Part model, mm, in its own coordinate system. A direction names the side the tool comes from. Round coordinates to 2 decimals unless told otherwise and drop trailing zeros. Write each loop counter-clockwise with the first axis right and the second up, starting at its lowest first coordinate (ties: lowest second). Pieces come first, ordered by that corner, then holes. Notation, with made-up numbers: M 83.25,48.5 L 108.25,48.5 A25 ccw 108.25,73.5 Z; hole C -26.5,0 d4. An arc over 180 degrees is marked long. Use one line per item in the form item = value. Start each with the question number.
Item 1: Cut at D-D, the plane z = 0. Give the cut face in (x, y).
Item 2: Cut at B-B, the plane z = -20.4. Give the cut face in (x, y).
Item 3: Which spindle directions (+Z, -Z, +X, -X, +Y, -Y) get a long thin tool onto all of the face, cutting with end or side? Do faces 1 (the face through (7.5, -17, -44)), 2 (the face through (-40, 0, 0)), 3 (the face through (40, 0, 0)), 4 (the face through (-43.7, 0.6, -20.9)), 5 (the face through (0, 0, 29)). Say none if no direction does.
Item 4: Mould opens along X. For faces 6 (the face through (38.9, 0.6, 19.6)), 7 (the face through (-1.352, 21.906, -4.292)), 8 (the face through (15, 0, -38)) say: +X half, -X half, draft (parallel to the pull), parting line (faces both ways), or undercut.
Item 5: Cut at A-A, the plane x = 41.35. Give the cut face in (y, z).
Item 6: Flat gauge pins, fed straight in: pin 1 Ø8 at (x, z) = (-41.25, -20.4) entering from -Y; pin 2 Ø20 at (y, z) = (-17, -44.5) entering from -X; pin 3 Ø8 at (x, z) = (-25.5, -3) entering from +Y; pin 4 Ø4.5 at (x, z) = (41.35, 20.1) entering from +Y. Where does each tip first touch, or does it go through?
Item 7: Cut at C-C, the plane x = 0. Give the cut face in (y, z), then the cut area to 3 significant figures.
Item 8: Probe L1, parallel to X at y = 0.6, z = -20.4; L2, parallel to Y at x = 9, z = -12.5; L3, parallel to Z at x = -12, y = -30. List the from-to ranges inside material, lowest first.
from build123d import *

# Parameters (mm, degrees)
SKETCH_1_W            = 95
SKETCH_1_H            = 53
EXTRUDE_244_DEPTH     = 1.2
CUT_EXTRUDE_624_REACH = 56.405
SKETCH_5_R            = 2.5
EXTRUDE_1004_DEPTH    = 35
SKETCH_7_R            = 4.5
EXTRUDE_1173_DEPTH    = 42


with BuildPart() as part:
    # 草图1 → Extrude 244 (new body)
    with BuildSketch(Plane(origin=(0, 0, 0), x_dir=(1, 0, 0), z_dir=(0, 1, 0))):
        Rectangle(SKETCH_1_W, SKETCH_1_H)
    extrude(amount=EXTRUDE_244_DEPTH)

    # 草图5 → Cut-Extrude 624 (cut, up to next)
    with BuildSketch(Plane(origin=(0, 1.2, 0), x_dir=(1, 0, 0), z_dir=(0, 1, 0)), mode=Mode.PRIVATE) as cut_extrude_624_sk1:
        with Locations(Location((-41.25, 20.4, 0), (0, 0, 270))):
            Circle(SKETCH_5_R)
    cut_extrude_624_tool1 = extrude(cut_extrude_624_sk1.sketch, amount=-CUT_EXTRUDE_624_REACH, mode=Mode.PRIVATE) & part.part
    # 草图5 → Cut-Extrude 624 (cut, up to next)
    with BuildSketch(Plane(origin=(0, 1.2, 0), x_dir=(1, 0, 0), z_dir=(0, 1, 0)), mode=Mode.PRIVATE) as cut_extrude_624_sk2:
        with Locations(Location((41.35, 20.4, 0), (0, 0, 270))):
            Circle(SKETCH_5_R)
    cut_extrude_624_tool2 = extrude(cut_extrude_624_sk2.sketch, amount=-CUT_EXTRUDE_624_REACH, mode=Mode.PRIVATE) & part.part
    # 草图5 → Cut-Extrude 624 (cut, up to next)
    with BuildSketch(Plane(origin=(0, 1.2, 0), x_dir=(1, 0, 0), z_dir=(0, 1, 0)), mode=Mode.PRIVATE) as cut_extrude_624_sk3:
        with Locations(Location((-41.25, -20.1, 0), (0, 0, 270))):
            Circle(SKETCH_5_R)
    cut_extrude_624_tool3 = extrude(cut_extrude_624_sk3.sketch, amount=-CUT_EXTRUDE_624_REACH, mode=Mode.PRIVATE) & part.part
    # 草图5 → Cut-Extrude 624 (cut, up to next)
    with BuildSketch(Plane(origin=(0, 1.2, 0), x_dir=(1, 0, 0), z_dir=(0, 1, 0)), mode=Mode.PRIVATE) as cut_extrude_624_sk4:
        with Locations(Location((41.35, -20.1, 0), (0, 0, 270))):
            Circle(SKETCH_5_R)
    cut_extrude_624_tool4 = extrude(cut_extrude_624_sk4.sketch, amount=-CUT_EXTRUDE_624_REACH, mode=Mode.PRIVATE) & part.part
    add(cut_extrude_624_tool1.solids().sort_by_distance((-41.25, 1.2, -20.4))[0], mode=Mode.SUBTRACT)
    add(cut_extrude_624_tool2.solids().sort_by_distance((41.35, 1.2, -20.4))[0], mode=Mode.SUBTRACT)
    add(cut_extrude_624_tool3.solids().sort_by_distance((-41.25, 1.2, 20.1))[0], mode=Mode.SUBTRACT)
    add(cut_extrude_624_tool4.solids().sort_by_distance((41.35, 1.2, 20.1))[0], mode=Mode.SUBTRACT)

    # 草图6 → Extrude 1004 (add)
    with BuildSketch(Plane.XZ):
        Polygon((32.5, -56.5), (7.5, -56.5), (7.5, -31.5), (-32.5, -31.5), (-32.5, 31.5), (32.5, 31.5), align=None)
    extrude(amount=EXTRUDE_1004_DEPTH)

    # 草图7 → Extrude 1173 (add)
    with BuildSketch(Plane(origin=(0, 1.2, 0), x_dir=(1, 0, 0), z_dir=(0, 1, 0))):
        with Locations(Location((0, 0, 0), (0, 0, 90))):
            Circle(SKETCH_7_R)
    extrude(amount=EXTRUDE_1173_DEPTH)


solid = part.part
Model answer:
q1.outline = M -47.5,0 L -32.5,0 L -32.5,-35 L 32.5,-35 L 32.5,0 L 47.5,0 L 47.5,1.2 L 4.5,1.2 L 4.5,43.2 L -4.5,43.2 L -4.5,1.2 L -47.5,1.2 Z
q2.outline = M -47.5,0 L -43.75,0 L -43.75,1.2 L -47.5,1.2 Z; M -38.75,0 L -32.5,0 L -32.5,-35 L 32.5,-35 L 32.5,0 L 38.85,0 L 38.85,1.2 L -38.75,1.2 Z; M 43.85,0 L 47.5,0 L 47.5,1.2 L 43.85,1.2 Z
q3.face_1 = -Z, -X, +Y, -Y
q3.face_2 = +Z, -Z, -X, -Y
q3.face_3 = +Z, -Z, +X, -Y
q3.face_4 = +Y, -Y
q3.face_5 = +Z, +X, -X, +Y
q4.face_6 = undercut
q4.face_7 = parting line
q4.face_8 = draft
q5.outline = M 0,-26.5 L 1.2,-26.5 L 1.2,-22.9 L 0,-22.9 Z; M 0,-17.9 L 1.2,-17.9 L 1.2,17.6 L 0,17.6 Z; M 0,22.6 L 1.2,22.6 L 1.2,26.5 L 0,26.5 Z
q6.pin_1 = 0
q6.pin_2 = 7.5
q6.pin_3 = 1.2
q6.pin_4 = through
q7.outline = M -35,-31.5 L 0,-31.5 L 0,-26.5 L 1.2,-26.5 L 1.2,-4.5 L 43.2,-4.5 L 43.2,4.5 L 1.2,4.5 L 1.2,26.5 L 0,26.5 L 0,31.5 L -35,31.5 Z
q7.area = 2,650 mm²
q8.L1 = -47.5 to -43.75, -38.75 to 38.85, 43.85 to 47.5
q8.L2 = -35 to 1.2
q8.L3 = -31.5 to 31.5
